Build history of the part. All positions in model axes, mm. A direction names the side the tool comes from. Give positions to 0.01 mm unless a question says otherwise; leave off trailing zeros. Loops run counter-clockwise (first coordinate to the right, second up) from the corner with the lowest first, then second, coordinate; pieces in that order, holes last. Notation, with made-up numbers: M 21,-17 L 29,-17 A26 cw 29,3 Z; hole C 11,77.5 d5. An arc over 180 degrees is marked long. Put each result on its own line as item: value.
Autodesk Inventor part; units mm, degrees
ref_plane "YZ Plane" through (0, 0, 0) normal (1, 0, 0) x (0, 1, 0)
ref_plane "XZ Plane" through (0, 0, 0) normal (0, 1, 0) x (-1, 0, 0)
ref_plane "XY Plane" through (0, 0, 0) normal (0, 0, 1) x (1, 0, 0)
sketch "Sketch1" plane through (0, 0, 0) normal (0, 1, 0) x (-1, 0, 0)
  circle A0 centre (0, 0) radius 17.25
  dimension "d0" = 34.5
extrude "Extrusion1" add sketch "Sketch1" along normal blind 74
sketch "Sketch2" plane through (0, 74, 0) normal (0, 1, 0) x (1, 0, 0)
  circle A0 centre (0, 0) radius 33.5
  dimension "d3" = 67
extrude "Extrusion2" add sketch "Sketch2" along normal blind 4
fillet "Fillet1" radius 13 1 edges at (17.25, 74, 0)
sketch "Sketch3" plane through (0, 78, 0) normal (0, 1, 0) x (1, 0, 0)
  circle A0 centre (0, 0) radius 13.75
  dimension "d8" = 27.5
extrude "Extrusion3" cut sketch "Sketch3" against normal blind 74
fillet "Fillet2" radius 13 1 edges at (-13.75, 78, 0)
fillet "Fillet3" radius 2 1 edges at (17.25, 0, 0)
properties part number "Juice_Extractor_Pusher"
Q1. Probe line 1 (Z direction, x = 0, y = 19); line 2 (Z direction, x = 11.5, y = 30); line 3 (X direction, y = 39.5, z = -4.5). List the from-to ranges inside material, lowest first. Write a range as from..to.
Here are the results:
line 1: -17.25..-13.75, 13.75..17.25
line 2: -12.86..-7.54, 7.54..12.86
line 3: -16.65..-12.99, 12.99..16.65
Q2. Slice it at A-A (z = 0). List the corners of the cut face in (x, y), and give its area (3 significant figures).
Here are the results:
outline: M -33.5,74 L -30.25,74 A13 cw -17.25,61 L -17.25,2 A2 ccw -15.25,0 L 15.25,0 A2 ccw 17.25,2 L 17.25,61 A13 cw 30.25,74 L 33.5,74 L 33.5,78 L 26.75,78 A13 ccw 13.75,65 L 13.75,4 L -13.75,4 L -13.75,65 A13 ccw -26.75,78 L -33.5,78 Z
area: 784 mm²
Q3. Tool access for faces 4 (the cylindrical face through (-2.981, 34.927, 13.423)), 5 (the flat face through (-25, 78, 10)), 6 (the cylindrical face through (-16.453, 31.087, -5.181)): list every direction of +Z, -Z, +X, -X, +Y, -Y with a clear straight run to the whole face (end or side of a thin tool).
Here are the results:
face 4: +Y
face 5: +Z, -Z, +X, -X, +Y
face 6: -Y
Q4. Mould opens along X. For faces 1 (the flat face through (-5, 74, -30)), 2 (the cylindrical face through (-7.262, 75.972, -32.703)), 3 (the flat face through (0, 4, 0)) say: pulls with the +X half, pulls with the -X half, needs draft (parallel to the pull), parting line crosses it, or undercut.
Here are the results:
face 1: needs draft
face 2: parting line crosses it
face 3: undercut
Q5. Slice it at D-D (y = 62.5). List the corners of the cut face in (x, z), and give its area (3 significant figures).
Here are the results:
outline: C 0,0 d34.67; hole C 0,0 d27.5
area: 350 mm²
Q6. Drop flat-ended pins along their axis: pin 1 Ø1.5 at (x, y) = (19.5, 28) entering from -Z; pin 2 Ø4 at (y, z) = (67, -13) entering from +X; pin 3 Ø4 at (x, y) = (2, 65) entering from -Z; pin 4 Ø22 at (x, z) = (-4, -1) entering from +Y. Give the stop position or say it passes through.
Here are the results:
pin 1: through
pin 2: x = 15.78
pin 3: z = -18.63
pin 4: y = 70.82
Q7. Slice it at C-C (y = 50.5). List the corners of the cut face in (x, z).
Here are the results:
outline: C 0,0 d34.5; hole C 0,0 d27.5
Q8. Slice it at B-B (x = 0). List the corners of the cut face in (y, z).
Here are the results:
outline: M 0,-15.25 A2 ccw 2,-17.25 L 61,-17.25 A13 cw 74,-30.25 L 74,-33.5 L 78,-33.5 L 78,-26.75 A13 ccw 65,-13.75 L 4,-13.75 L 4,13.75 L 65,13.75 A13 ccw 78,26.75 L 78,33.5 L 74,33.5 L 74,30.25 A13 cw 61,17.25 L 2,17.25 A2 ccw 0,15.25 Z
